Geometry check sheet. Reference: the model listing, model coordinates, mm. Give positions to 0.01 mm unless a question says otherwise; leave off trailing zeros. Write each loop counter-clockwise with the first axis right and the second up, starting at its lowest first coordinate (ties: lowest second). Pieces come first, ordered by that corner, then holes. Notation, with made-up numbers: (28.5, 21.5) - (77.5, 21.5) arc R28 cw to (77.5, 59.5) - close; hole circle Ø11 at (-3, -31). An arc over 180 degrees is marked (long way). Write item = value, one per line. Start each with the question number.
(1) Thickness scan on L1, parallel to Y at x = 275.5, z = 2.25; L2, parallel to X at y = 104.5, z = 2; L3, parallel to X at y = 136.5, z = 1.5. Record the ranges inside material, lowest first.
(2) Section check C-C, the plane y = 157. Enter the section's corners in (x, z) (3 decimals), plus the area to 3 significant figures.
(3) Section check A-A, the plane z = 2. Give the number of separate pieces and of enclosed holes in the cut face, plus the area to 3 significant figures.
(4) Depth check by flat-ended pin: pin 1 Ø2 at (x, z) = (328, 5) entering from -Y; pin 2 Ø9 at (x, y) = (193.675, 254) entering from -Z; pin 3 Ø6 at (x, y) = (496.89, 60.92) entering from +Z; pin 4 Ø1.5 at (x, z) = (128, 2.5) entering from +Y. Enter the tip coordinate at first touch or a pass-through.
(5) Section check B-B, the plane x = 126.5. Enter the section's corners in (y, z) (3 decimals).
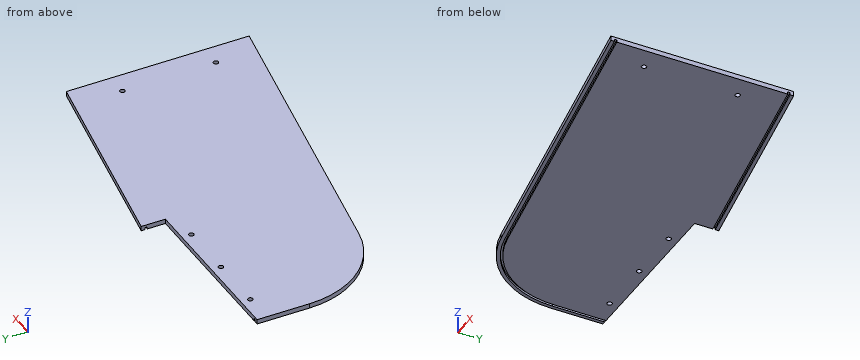
Autodesk Inventor part; units mm, degrees
ref_plane "YZ Plane" through (0, 0, 0) normal (1, 0, 0) x (0, 1, 0)
ref_plane "XZ Plane" through (0, 0, 0) normal (0, 1, 0) x (-1, 0, 0)
ref_plane "XY Plane" through (0, 0, 0) normal (0, 0, 1) x (1, 0, 0)
sketch "Sketch1" plane through (0, 0, 0) normal (0, 0, 1) x (1, 0, 0)
  line L0 (0, 0) -> (236.5375, 0)
  line L1 (527.05, 0) -> (527.05, 248.2464)
  line L2 (236.5375, 266.7) -> (0, 266.7)
  line L3 (0, 266.7) -> (0, 195.5132)
  line L4 (527.05, 0) -> (101.0217, 75.1203)
  line L5 (527.05, 248.2464) -> (236.5375, 299.4716)
  line L6 (236.5375, 266.7) -> (236.5375, 299.4716)
  arc A0 (0, 195.5132) -> (101.0217, 75.1203) centre (122.2502, 195.5132) ccw
  circle A1 centre (496.8875, 187.9214) radius 3.3655
  circle A2 centre (496.8875, 60.9214) radius 3.3655
  point P0 (0, 92.9331)
  dimension "d0" = 266.7
  dimension "d2" = 10
  dimension "d3" = 244.475
  dimension "d4" = 236.5375
  dimension "d5" = 527.05
  dimension "d18" = 122.2502
  dimension "d20" = 6.731
  dimension "d21" = 60.325
  dimension "d22" = 127
  dimension "d23" = 30.1625
  dimension "d24" = 30.1625
extrude "Extrusion1" add sketch "Sketch1" along normal blind 6.35 contours L4 A0 L3 L2 L6 L5 L1 | A1 | A2
sketch "Sketch2" plane through (0, 0, 0) normal (0, 0, -1) x (-1, 0, 0)
  line L0 (-527.05, 248.2464) -> (-236.5375, 299.4716)
  line L1 (-101.0217, 75.1203) -> (-527.05, 0)
  arc A0 (-101.0217, 75.1203) -> (0, 195.5132) centre (-122.2502, 195.5132) ccw
  line L2 (0, 266.7) -> (0, 195.5132)
  line L3 (-527.05, 243.4105) -> (-236.5375, 294.6356)
  line L4 (-527.05, 240.1865) -> (-236.5375, 291.4117)
  line L5 (-527.05, 4.836) -> (-101.8487, 79.8104)
  arc A1 (-101.8487, 79.8104) -> (-4.7625, 195.5132) centre (-122.2502, 195.5132) ccw
  line L6 (-4.7625, 195.5132) -> (-4.7625, 266.7)
  line L7 (-527.05, 8.0599) -> (-102.4, 82.9372)
  arc A2 (-102.4, 82.9372) -> (-7.9375, 195.5132) centre (-122.2502, 195.5132) ccw
  line L8 (-7.9375, 195.5132) -> (-7.9375, 266.7)
  line L9 (-527.05, 0) -> (-527.05, 248.2464)
  line L10 (-236.5375, 299.4716) -> (-236.5375, 266.7)
  line L11 (-236.5375, 266.7) -> (0, 266.7)
  line L12 (-527.05, 240.1865) -> (-527.05, 243.4105)
  line L13 (-236.5375, 294.6356) -> (-236.5375, 291.4117)
  line L14 (-7.9375, 266.7) -> (-4.7625, 266.7)
  line L15 (-527.05, 8.0599) -> (-527.05, 4.836)
  dimension "d27" = 4.7625
  dimension "d28" = 3.175
  dimension "d29" = 4.7625
  dimension "d30" = 4.7625
  dimension "d31" = 3.175
  dimension "d32" = 3.175
extrude "Extrusion2" cut sketch "Sketch2" against normal blind 3.175 contours L3 L10 L4 L9 | L7 A2 L8 L11 L6 A1 L5 L9
extrude "Extrusion3" cut sketch "Sketch1" along normal blind 25.4 contours A1 | A2
hole "Hole1" at (41.275, 254, 0) direction (0, 0, 1) diameter 6.731 depth 25.4 tip angle 118
pattern_linear "Rectangular Pattern1" count 3 spacing 76.2 along (1, 0, 0) of "Hole1"
equation "\"d24\" = d23"
equation "\"d29\" = d27"
equation "\"d30\" = d27"
properties part number "GE-12087-01"
Model answer:
q1.L1 = 44.36 to 49.19, 52.41 to 284.54, 287.77 to 292.6
q1.L2 = 40.63 to 47.95, 53.08 to 527.05
q1.L3 = 15.19 to 20.66, 24.35 to 527.05
q2.outline = (6.225, 0) - (11.254, 0) - (11.254, 3.175) - (14.621, 3.175) - (14.621, 0) - (527.05, 0) - (527.05, 6.35) - (6.225, 6.35) - close
q2.area = 3,300 mm²
q3.separate_pieces = 3
q3.enclosed_holes = 5
q3.area = 113,000 mm²
q4.pin_1 = 34.92
q4.pin_2 = 0
q4.pin_3 = through
q4.pin_4 = 266.7
q5.outline = (70.628, 0) - (75.464, 0) - (75.464, 3.175) - (78.688, 3.175) - (78.688, 0) - (266.7, 0) - (266.7, 6.35) - (70.628, 6.35) - close
